Job drawing, mm, ordinate dimensions from the low corner. One solid piece. A direction names the side the tool comes from. Give positions to 0.01 mm unless a question says otherwise; leave off trailing zeros. Loops run counter-clockwise (first coordinate to the right, second up) from the corner with the lowest first, then second, coordinate; pieces in that order, holes last. Notation, with made-up numbers: M 15,-3.75 L 68,-3.75 A24 ccw 68,29.25 Z; hole C -27,79.25 d8. An arc over 180 degrees is marked long. Answer as CSV lines item,"result".
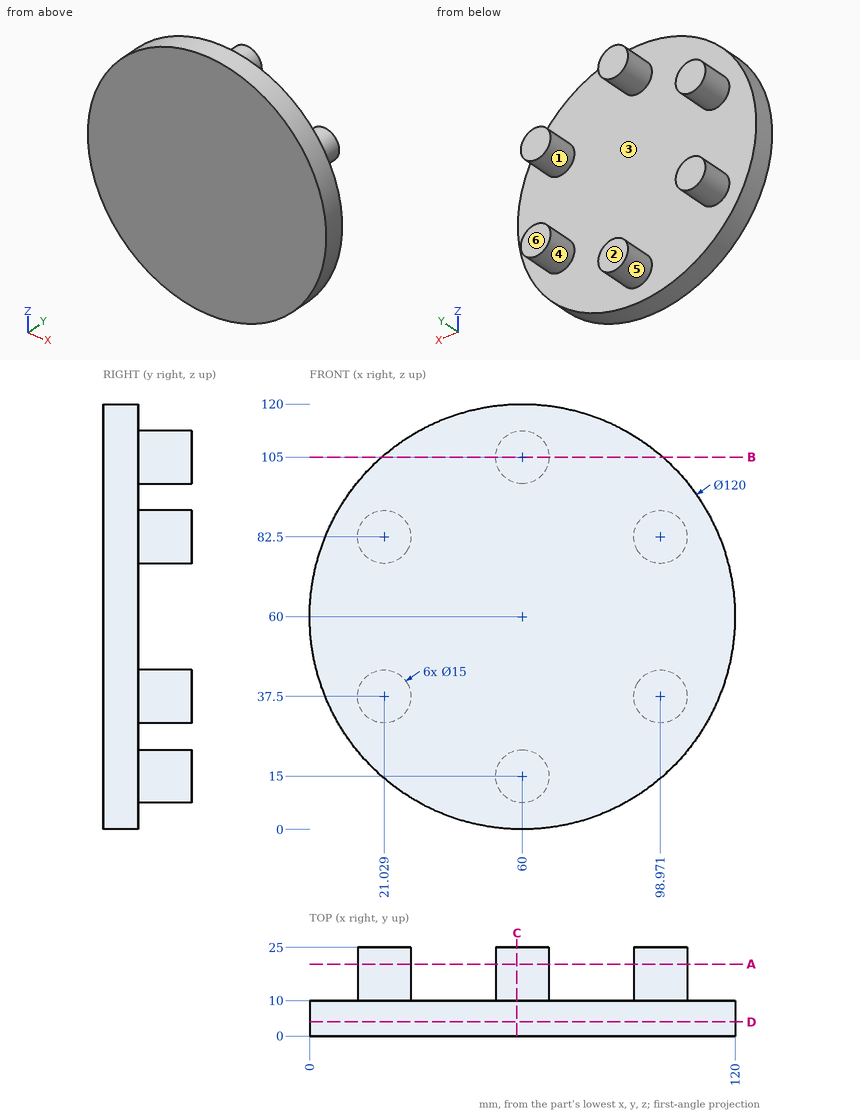
1) Mould opens along X. For the marked faces 3, 4, 5 and 6 say: +X half, -X half, draft (parallel to the pull), parting line (faces both ways), or undercut.
Answer below:
face 3,"undercut"
face 4,"undercut"
face 5,"parting line"
face 6,"draft"
2) Band-saw the part on A-A on y = 20.25. Give the cut face in (x, z), and give its area (3 significant figures).
Answer below:
outline,"C 21.03,37.5 d15; C 21.03,82.5 d15; C 60,15 d15; C 60,105 d15; C 98.97,37.5 d15; C 98.97,82.5 d15"
area,"1,060 mm^2"
3) Flat gauge pins, fed straight in: pin 1 (12 mm diameter, centred on y = 18, z = 95, fed in from -X); pin 2 (1.5 mm diameter, centred on x = 87.5, y = 9, fed in from +Z); pin 3 (3 mm diameter, centred on y = 9.5, z = 102.5, fed in from +X); pin 4 (1 mm diameter, centred on x = 22, z = 33, fed in from -Y). Where does each tip first touch, or does it go through?
Answer below:
pin 1,"stops at x = 17.29"
pin 2,"stops at z = 113.71"
pin 3,"stops at x = 103.81"
pin 4,"stops at y = 0"
4) Band-saw the part on C-C on x = 58.5. Give the cut face in (y, z).
Answer below:
outline,"M 0,0.02 L 10,0.02 L 10,7.65 L 25,7.65 L 25,22.35 L 10,22.35 L 10,97.65 L 25,97.65 L 25,112.35 L 10,112.35 L 10,119.98 L 0,119.98 Z"
5) Which spindle directions (+Z, -Z, +X, -X, +Y, -Y) get a long thin tool onto all of the face, cutting with end or side? Do the marked faces 1 and 2. Say none if no direction does.
Answer below:
face 1,"+Y"
face 2,"+Z, -Z, +X, -X, +Y"
6) Drill centre lines: line 1 (Y direction, x = 84, z = 101); line 2 (X direction, y = 17.25, z = 82.5); line 3 (X direction, y = 16, z = 81.5). Where is each one in solid material? Low to high. Write a range as from..to.
Answer below:
line 1,"y = 0..10"
line 2,"x = 13.53..28.53, 91.47..106.47"
line 3,"x = 13.6..28.46, 91.54..106.4"
7) Band-saw the part on D-D on y = 4. Give the cut face in (x, z).
Answer below:
outline,"C 60,60 d120"
8) Band-saw the part on B-B on z = 105. Give the cut face in (x, y), and give its area (3 significant figures).
Answer below:
outline,"M 20.31,0 L 99.69,0 L 99.69,10 L 67.5,10 L 67.5,25 L 52.5,25 L 52.5,10 L 20.31,10 Z"
area,"1,020 mm^2"
